Geometry check sheet. Reference: the model listing, model coordinates, mm. Face numbers are marked on the shaded views. A direction names the side the tool comes from. Round coordinates to 2 decimals unless told otherwise and drop trailing zeros. Order: outer loops, then holes, each group sorted by start corner. A loop starts at its lowest first (then second) coordinate and runs counter-clockwise, first axis right, second up. Notation, with made-up numbers: (-11, 68) - (33, 68) arc R9 cw to (33, 84) - close; hole circle Ø10 at (-17, -29). An arc over 180 degrees is marked (long way). Use a Markdown table: item, result. Add a question column.
(1) Section check C-C on x = -14. Record the boundary of the cut face in (y, z), then the cut area to 3 significant figures.
(2) Access from +Z, -Z, +X, -X, +Y, -Y to the whole of each face (thin tool, end or side, straight path). Record for the marked faces 1, 2 and 3.
(3) Thickness scan on line 1 along X through (y, z) = (0.5, 2); line 2 along X through (y, z) = (18, 0.25); line 3 along Y through (x, z) = (12, 3.75). Record the ranges inside material, lowest first. Write a range as [from, to].
(4) Mould release check, pull along X, two halves, no side actions. Record for the marked faces 4, 5, 6 and 7: released by +X, released by -X, zero draft, split by the parting line, or undercut.
(5) Section check D-D on y = 7.75. Record the boundary of the cut face in (x, z).
(6) Section check A-A on y = 1.25. Record the boundary of the cut face in (x, z), then the cut area to 3 significant figures.
(7) Gauge pin test, flat ends, axial feed: P1, Ø8, axis at x = -6.5, z = -2, coming from the +Y side; P2, Ø5, axis at x = 5.5, z = -6.5, coming from the +Y side; P3, Ø4, axis at x = 13.5, y = 6, coming from the +Z side; P4, Ø3, axis at x = -1, y = -6, coming from the +Z side. Record the tip position at first contact, or that the pin passes through.
(8) Section check B-B on z = -7.5. Record the boundary of the cut face in (x, y).
```python
from build123d import *

# Parameters (mm, degrees)
SKETCH1_W                = 25
SKETCH1_H                = 21
BOSS_EXTRUDE1_DEPTH      = 11
SKETCH2_W                = 25
SKETCH2_H                = 1
BOSS_EXTRUDE2_DEPTH      = 10
BOSS_EXTRUDE3_DEPTH      = 10
SKETCH4_W                = 30.5
SKETCH4_H                = 25
BOSS_EXTRUDE4_DEPTH      = 1.5
BOSS_EXTRUDE5_DEPTH      = 8.5
BOSS_EXTRUDE5_DEPTH_BACK = 8.5


with BuildPart() as part:
    # Sketch1 → Boss-Extrude1 (new body)
    with BuildSketch(Plane(origin=(0, 0, 0), x_dir=(1, 0, 0), z_dir=(0, 1, 0))):
        Rectangle(SKETCH1_W, SKETCH1_H)
    extrude(amount=BOSS_EXTRUDE1_DEPTH)

    # Sketch2 → Boss-Extrude2 (add)
    with BuildSketch(Plane(origin=(0, 11, 0), x_dir=(1, 0, 0), z_dir=(0, 1, 0))):
        Rectangle(SKETCH2_W, SKETCH2_H)
    extrude(amount=BOSS_EXTRUDE2_DEPTH)

    # Sketch3 → Boss-Extrude3 (add, symmetric)
    with BuildSketch(Plane.XY):
        Polygon((-12.5, 11), (-16.271420935, 3.81152577), (-16.271420935, 0.178717712), (-15.621420935, 0.178717712), (-15.621420935, 3.651367103), (-12.5, 9.600916182), align=None)
    boss_extrude3 = extrude(amount=BOSS_EXTRUDE3_DEPTH, both=True)

    # Mirror1: Boss-Extrude3 across plane
    add(boss_extrude3.mirror(Plane(origin=(0, 0, 0), x_dir=(0, 0, 1), z_dir=(1, 0, 0))))

    # Sketch4 → Boss-Extrude4 (add)
    with BuildSketch(Plane.XZ):
        Rectangle(SKETCH4_W, SKETCH4_H)
    extrude(amount=BOSS_EXTRUDE4_DEPTH)

    # Sketch5 → Boss-Extrude5 (add, two sides: drawn at the far end of the back side and taken through both)
    with BuildSketch(Plane.XY.offset(-BOSS_EXTRUDE5_DEPTH_BACK)):
        with BuildLine():
            Line((11.75, -1.5), (-11.75, -1.5))
            ThreePointArc((-11.75, -1.5), (-2.707390064, -3.962204019), (5.75, -8))
            ThreePointArc((5.75, -8), (9.254540353, -5.215729557), (11.75, -1.5))
        make_face()
    extrude(amount=BOSS_EXTRUDE5_DEPTH + BOSS_EXTRUDE5_DEPTH_BACK)


solid = part.part
```
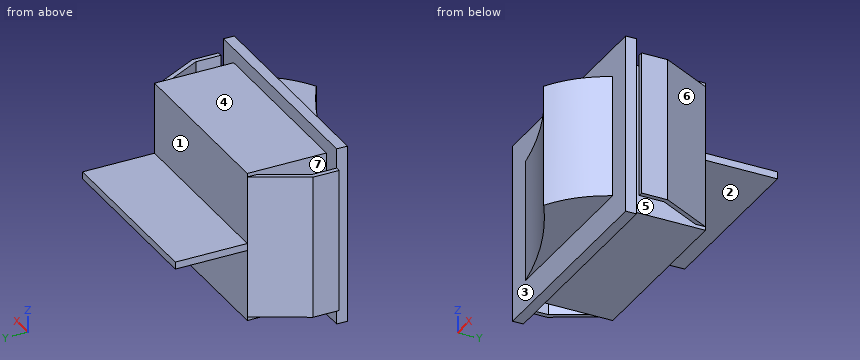
Check sheet entries:
| question | item | result |
|---|---|---|
| 1 | outline | (-1.5, -12.5) - (0, -12.5) - (0, 12.5) - (-1.5, 12.5) - close; (6.74, -10) - (8.14, -10) - (8.14, 10) - (6.74, 10) - close |
| 1 | area | 65.5 mm2 |
| 2 | face 1 | +Z, +X, -X, +Y |
| 2 | face 2 | -Z, +X, -X, +Y |
| 2 | face 3 | -Y |
| 3 | line 1 | x = [-16.27, -15.62], [-12.5, 12.5], [15.62, 16.27] |
| 3 | line 2 | x = [-12.5, 12.5] |
| 3 | line 3 | y = [-1.5, 11] |
| 4 | face 4 | zero draft |
| 4 | face 5 | undercut |
| 4 | face 6 | released by +X |
| 4 | face 7 | undercut |
| 5 | outline | (-14.21, -10) - (-13.47, -10) - (-13.47, 10) - (-14.21, 10) - close; (-12.5, -10.5) - (12.5, -10.5) - (12.5, 10.5) - (-12.5, 10.5) - close; (13.47, -10) - (14.21, -10) - (14.21, 10) - (13.47, 10) - close |
| 6 | outline | (-16.27, -10) - (-15.62, -10) - (-15.62, 10) - (-16.27, 10) - close; (-12.5, -10.5) - (12.5, -10.5) - (12.5, 10.5) - (-12.5, 10.5) - close; (15.62, -10) - (16.27, -10) - (16.27, 10) - (15.62, 10) - close |
| 6 | area | 551 mm2 |
| 7 | P1 | stops at y = 21 |
| 7 | P2 | stops at y = 11 |
| 7 | P3 | stops at z = 10.5 |
| 7 | P4 | stops at z = 8.5 |
| 8 | outline | (-16.27, 0.18) - (-15.62, 0.18) - (-15.62, 3.65) - (-12.5, 9.6) - (-12.5, 0) - (-15.25, 0) - (-15.25, -1.5) - (-11.75, -1.5) arc R52.26 cw to (5.75, -8) arc R14.59 ccw to (11.75, -1.5) - (15.25, -1.5) - (15.25, 0) - (12.5, 0) - (12.5, 9.6) - (15.62, 3.65) - (15.62, 0.18) - (16.27, 0.18) - (16.27, 3.81) - (12.5, 11) - (-12.5, 11) - (-16.27, 3.81) - close |
